For this review, take the finished solid that the model builds, in its own axes (mm). Face numbers are marked on the shaded views. A direction names the side the tool comes from. Round coordinates to 2 decimals unless told otherwise and drop trailing zeros. Write each loop counter-clockwise with the first axis right and the second up, starting at its lowest first coordinate (ties: lowest second). Pieces come first, ordered by that corner, then holes. Notation, with made-up numbers: M -32,-14.75 L -10,-14.75 A10 cw -10,-5.75 Z; hole C 49.25,62.5 d2. An arc over 180 degrees is marked long. One line per question, with ' | ' between items.
```python
from build123d import *

# Parameters (mm, degrees)
EXTRUDE_1_DEPTH     = 19
CUT_EXTRUDE_2_DEPTH = 43
CUT_EXTRUDE_3_DEPTH = 2
EXTRUDE_2_DEPTH     = 14
SKETCH_5_R          = 2.48
EXTRUDE_3_DEPTH     = 2
CUT_EXTRUDE_4_DEPTH = 50
EXTRUDE_START       = 2
SKETCH_7_R          = 2.48
EXTRUDE_4_DEPTH     = 2
SKETCH_8_W          = 1.371307674
SKETCH_8_H          = 2.48
EXTRUDE_5_DEPTH     = 2
CUT_EXTRUDE_5_DEPTH = 10
CUT_EXTRUDE_6_DEPTH = 2
SKETCH_11_W         = 2.08463024
SKETCH_11_H         = 2.48
EXTRUDE_7_DEPTH     = 2
CUT_EXTRUDE_7_DEPTH = 20
CUT_EXTRUDE_8_DEPTH = 2.5
CUT_EXTRUDE_9_DEPTH = 50


with BuildPart() as part:
    # 草图1 → 凸台-拉伸1 (new body)
    with BuildSketch(Plane.XY):
        with BuildLine():
            Line((0, 0), (7, 0))
            Line((7, 0), (7, -5))
            ThreePointArc((7, -5), (7.25, -5.25), (7, -5.5))
            Line((7, -5.5), (7, -9))
            Line((7, -9), (9, -9))
            Line((9, -9), (7, -13))
            Line((7, -13), (7, -45))
            Line((7, -45), (0, -45))
            Line((0, -45), (-7, -45))
            Line((-7, -45), (-7, -13))
            Line((-7, -13), (-9, -9))
            Line((-9, -9), (-7, -9))
            Line((-7, -9), (-7, -5.5))
            ThreePointArc((-7, -5.5), (-7.25, -5.25), (-7, -5))
            Line((-7, -5), (-7, 0))
            Line((-7, 0), (0, 0))
        make_face()
    extrude(amount=EXTRUDE_1_DEPTH)

    # 草图2 → 切除-拉伸2 (cut)
    with BuildSketch(Plane(origin=(0, 0, 0), x_dir=(1, 0, 0), z_dir=(0, 1, 0))):
        Polygon((0, -2), (5, -2), (5, -9.5), (5, -17), (0, -17), (-5, -17), (-5, -9.5), (-5, -2), align=None)
    extrude(amount=-CUT_EXTRUDE_2_DEPTH, mode=Mode.SUBTRACT)

    # 草图3 → 切除-拉伸3 (cut)
    with BuildSketch(Plane.XY.offset(19)):
        Polygon((0, -23), (5, -23), (5, -43), (0, -43), (-5, -43), (-5, -23), align=None)
    extrude(amount=-CUT_EXTRUDE_3_DEPTH, mode=Mode.SUBTRACT)

    # 草图4 → 凸台-拉伸2 (add)
    with BuildSketch(Plane.XY.offset(19)):
        Polygon((-7, -42.996240591), (-7, -45), (7, -45), (7, -42.996240591), (5, -42.996240591), (5, -43), (-5, -43), (-5, -42.996240591), align=None)
        Polygon((-7, -23), (5, -23), (7, -23), (7, -21), (-7, -21), align=None)
    extrude(amount=EXTRUDE_2_DEPTH)

    # 草图5 → 凸台-拉伸3 (add)
    with BuildSketch(Plane.XZ.offset(45)):
        with Locations(Location((0, 26, 0), (0, 0, 270))):
            Circle(SKETCH_5_R)
    extrude(amount=EXTRUDE_3_DEPTH)

    # 草图6 → 切除-拉伸4 (cut)
    with BuildSketch(Plane(origin=(0, -45, 0), x_dir=(-1, 0, 0), z_dir=(0, -1, 0))):
        with BuildLine():
            Line((7, -33), (7, -26))
            ThreePointArc((7, -26), (4.949747468, -30.949747468), (0, -33))
            Line((0, -33), (7, -33))
        make_face()
        with BuildLine():
            Line((-7, -33), (0, -33))
            ThreePointArc((0, -33), (-4.949747468, -30.949747468), (-7, -26))
            Line((-7, -26), (-7, -33))
        make_face()
    extrude(amount=-CUT_EXTRUDE_4_DEPTH, mode=Mode.SUBTRACT)

    # 草图7 → 凸台-拉伸4 (add)
    with BuildSketch(Plane(origin=(0, -21, 0), x_dir=(1, 0, 0), z_dir=(0, 1, 0)).offset(EXTRUDE_START)):
        with Locations(Location((0, -26, 0), (0, 0, 90))):
            Circle(SKETCH_7_R)
    extrude(amount=-EXTRUDE_4_DEPTH)

    # 草图8 → 凸台-拉伸5 (add)
    with BuildSketch(Plane(origin=(0, -21, 0), x_dir=(1, 0, 0), z_dir=(0, 1, 0))):
        with Locations((4.228560023, -27.24)):
            Rectangle(SKETCH_8_W, SKETCH_8_H)
    extrude(amount=EXTRUDE_5_DEPTH)

    # 草图9 → 切除-拉伸5 (cut)
    with BuildSketch(Plane(origin=(4.91421386, 0, 0), x_dir=(0, 0, -1), z_dir=(1, 0, 0))):
        Polygon((-26, -19), (-28.48, -19), (-28.48, -20), align=None)
    extrude(amount=-CUT_EXTRUDE_5_DEPTH, mode=Mode.SUBTRACT)

    # 草图10 → 切除-拉伸6 (cut)
    with BuildSketch(Plane(origin=(4.91421386, 0, 0), x_dir=(0, 0, -1), z_dir=(1, 0, 0))):
        Polygon((-26, -19), (-26, -21), (-28.48, -21), (-28.48, -20), align=None)
    extrude(amount=-CUT_EXTRUDE_6_DEPTH, mode=Mode.SUBTRACT)

    # 草图11 → 凸台-拉伸7 (add)
    with BuildSketch(Plane(origin=(0, -47, 0), x_dir=(-1, 0, 0), z_dir=(0, -1, 0))):
        with Locations((-4.196152556, -27.25184449)):
            Rectangle(SKETCH_11_W, SKETCH_11_H)
    extrude(amount=-EXTRUDE_7_DEPTH)

    # 草图12 → 切除-拉伸7 (cut)
    with BuildSketch(Plane(origin=(5.238467676, 0, 0), x_dir=(0, 0, -1), z_dir=(1, 0, 0))):
        Polygon((-28.49184449, -47), (-28.49184449, -46), (-26.01184449, -47), align=None)
    extrude(amount=-CUT_EXTRUDE_7_DEPTH, mode=Mode.SUBTRACT)

    # 草图13 → 切除-拉伸8 (cut)
    with BuildSketch(Plane(origin=(5.238467676, 0, 0), x_dir=(0, 0, -1), z_dir=(1, 0, 0))):
        Polygon((-28.49184449, -46), (-26.01184449, -47), (-26, -45), (-28.49184449, -45), align=None)
    extrude(amount=-CUT_EXTRUDE_8_DEPTH, mode=Mode.SUBTRACT)

    # 草图14 → 切除-拉伸9 (cut)
    with BuildSketch(Plane.XZ.offset(45)):
        with BuildLine():
            ThreePointArc((1.5, 32.837397166), (0.754393744, 32.959230567), (0, 33))
            Line((0, 33), (0, 30))
            Line((0, 30), (1.5, 30))
            Line((1.5, 30), (1.5, 32.837397166))
        make_face()
        with BuildLine():
            Line((0, 30), (0, 33))
            ThreePointArc((0, 33), (-0.754393744, 32.959230567), (-1.5, 32.837397166))
            Line((-1.5, 32.837397166), (-1.5, 30))
            Line((-1.5, 30), (0, 30))
        make_face()
        with BuildLine():
            ThreePointArc((-1.5, 32.837397166), (-0.754393744, 32.959230567), (0, 33))
            ThreePointArc((0, 33), (0.754393744, 32.959230567), (1.5, 32.837397166))
            Line((1.5, 32.837397166), (1.5, 33.175350271))
            Line((1.5, 33.175350271), (-1.5, 33.175350271))
            Line((-1.5, 33.175350271), (-1.5, 32.837397166))
        make_face()
    extrude(amount=-CUT_EXTRUDE_9_DEPTH, mode=Mode.SUBTRACT)


solid = part.part
```
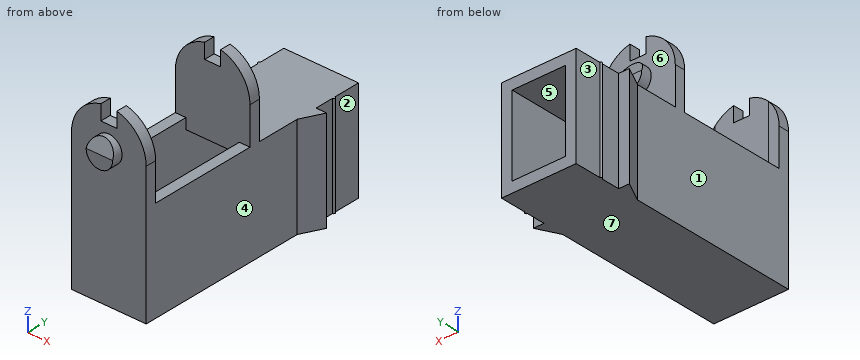
Item 1: Take a section at C-C (y = -8). Write out the cut boundary in (x, z), then the cut area to 3 significant figures.
Results:
outline: M -7,0 L 7,0 L 7,19 L -7,19 Z; hole M -5,2 L 5,2 L 5,17 L -5,17 Z | area: 116 mm2
Item 2: To check wall thickness, follow line 1 along Z through (x, y) = (-0.25, -16.5); line 2 along Y through (x, z) = (2.75, 29); line 3 along X through (y, z) = (-23, 5). State the ranges of each line that lie inside material, in increasing order. Write a range as from..to.
Results:
line 1: 0..2, 17..19 | line 2: -45..-43, -23..-21 | line 3: -7..-5, 5..7
Item 3: Take a section at A-A (z = 17.5). Write out the cut boundary in (x, y).
Results:
outline: M -9,-9 L -7,-13 L -7,-45 L 7,-45 L 7,-13 L 9,-9 L 7,-9 L 7,-5.5 A0.25 ccw 7,-5 L 7,0 L -7,0 L -7,-5 A0.25 ccw -7,-5.5 L -7,-9 Z; hole M -5,-43 L 5,-43 L 5,-23 L -5,-23 Z
Item 4: Mouldability with a two-part tool opening along Z and no side actions: class the marked faces 4, 5, 6 and 7 as +Z half, -Z half, draft (parallel to the pull), parting line (faces both ways), or undercut.
Results:
face 4: draft | face 5: undercut | face 6: undercut | face 7: -Z half
Item 5: Machinability: for the marked faces 1, 2 and 3, which of the approach directions +Z, -Z, +X, -X, +Y, -Y give a long, thin tool a straight path to every point of the face, cutting with its end or side? Answer none if there is none.
Results:
face 1: +Z, -Z, -X, -Y | face 2: +Z, -Z, +X, +Y | face 3: +Z, -Z, -X, +Y
Item 6: Insertion check: pin 1 Ø1 at (x, y) = (-6, -34) entering from +Z; pin 2 Ø2 at (x, z) = (8.5, 12) entering from +Y; pin 3 Ø1.6 at (y, z) = (-22.5, 31.5) entering from -X; pin 4 Ø1.5 at (y, z) = (-17, 27) entering from -X. Each pin has a flat end and moves straight along its axis. Give the tip position at first contact, or say it passes through.
Results:
pin 1: z = 19 | pin 2: y = -9 | pin 3: x = -5.19 | pin 4: through
Item 7: Take a section at B-B (x = 0). Write out the cut boundary in (y, z).
Results:
outline: M -47,23.52 L -45,23.52 L -45,0 L 0,0 L 0,2 L -43,2 L -43,30 L -45,30 L -45,28.48 L -46,28.48 L -47,26.01 Z; M -23,17 L 0,17 L 0,19 L -21,19 L -21,23.52 L -19,23.52 L -19,26 L -20,28.48 L -21,28.48 L -21,30 L -23,30 Z
